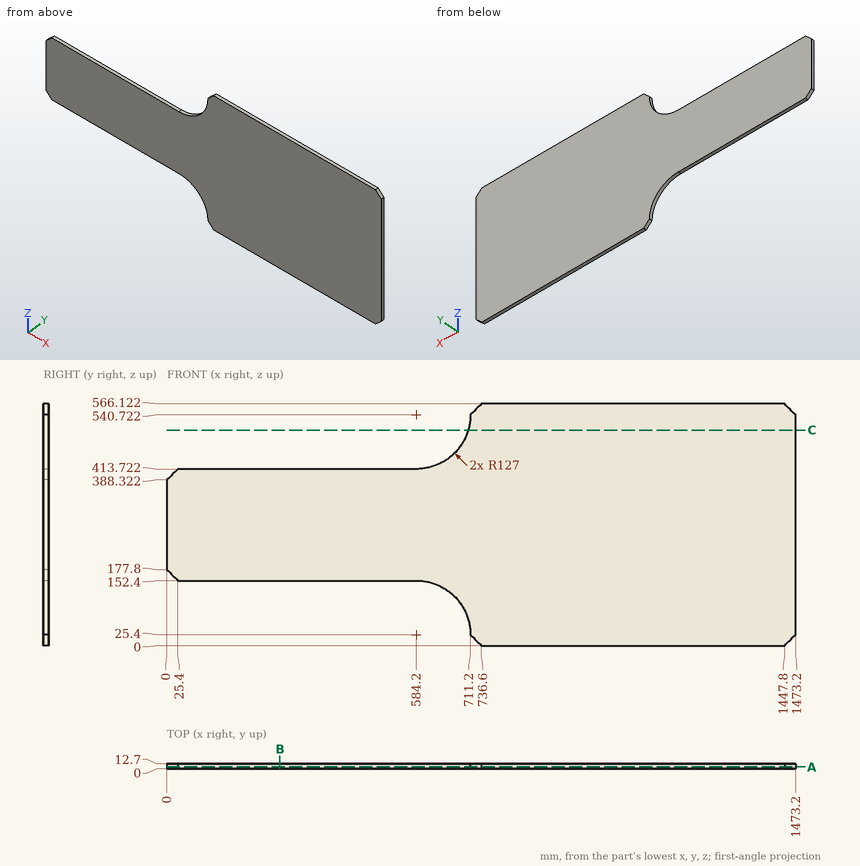
Here's the drawing with two shaded views (mm, measured from the low corner). I have some questions. Give positions to 0.01 mm unless a question says otherwise; leave off trailing zeros. Loops run counter-clockwise (first coordinate to the right, second up) from the corner with the lowest first, then second, coordinate; pieces in that order, holes last. Notation, with made-up numbers: (33, -2.5) -> (66, -2.5) arc R24 ccw to (66, 14.5) -> close; hole circle Ø1 at (-2, 67). An arc over 180 degrees is marked (long way). Answer as a JSON object with one key per item and string values. Group by question number.
Item 1: I need wall thicknesses on L1, parallel to Z at x = 93, y = 5.5; L2, parallel to X at y = 6.5, z = 505.5; L3, parallel to X at y = 7.5, z = 59.5 (1 decimal). Which ranges of each line are inside material? Lowest first, please.
Item 2: Imagine slicing it at A-A on y = 5. Write out the boundary of the cut face in (x, z), then the cut area to 3 significant figures.
Item 3: Will these pins go through, and if not, where does the flat tip stop? pin 1 (5 mm diameter, centred on x = 644, y = 8.5, fed in from +Z); pin 2 (6 mm diameter, centred on x = 408.5, y = 4.5, fed in from +Z); pin 3 (2 mm diameter, centred on x = 656.5, y = 4.5, fed in from -Z).
Item 4: Imagine slicing it at B-B on x = 265. Write out the boundary of the cut face in (y, z).
Item 5: Imagine slicing it at C-C on z = 505. Write out the boundary of the cut face in (x, y), then the cut area to 3 significant figures.
Answer list:
{
 "1": {"L1": "z = 152.4 to 413.72", "L2": "x = 706.22 to 1473.2", "L3": "x = 706.5 to 1473.2"},
 "2": {"outline": "(0, 177.8) -> (25.4, 152.4) -> (584.2, 152.4) arc R127 cw to (711.2, 25.4) -> (736.6, 0) -> (1447.8, 0) -> (1473.2, 25.4) -> (1473.2, 540.72) -> (1447.8, 566.12) -> (736.6, 566.12) -> (711.2, 540.72) arc R127 cw to (584.2, 413.72) -> (25.4, 413.72) -> (0, 388.32) -> close", "area": "622,000 mm2"},
 "3": {"pin 1": "stops at z = 430.05", "pin 2": "stops at z = 413.72", "pin 3": "stops at z = 129.11"},
 "4": {"outline": "(0, 152.4) -> (12.7, 152.4) -> (12.7, 413.72) -> (0, 413.72) -> close"},
 "5": {"outline": "(706.07, 0) -> (1473.2, 0) -> (1473.2, 12.7) -> (706.07, 12.7) -> close", "area": "9,740 mm2"}
}
